The listing builds one solid part. Answer for the finished solid, in the listing's coordinates (mm). A direction names the side the tool comes from. Coordinates: 2 decimals unless noted, no trailing zeros. Loops run counter-clockwise (first coordinate to the right, second up) from the corner with the lowest first, then second, coordinate; pieces in that order, holes last. Notation, with made-up numbers: M 20.25,-18 L 68.25,-18 A19 cw 68.25,-5 Z; hole C 16,-36.75 d10. An arc over 180 degrees is marked long. Answer in a Markdown table with one row per item. Add a question column.
from build123d import *

# Parameters (mm, degrees)
F1_DEPTH = 83.312


with BuildPart() as f1:
    # F0 (on Top) → F1 (new body)
    with BuildSketch(Plane.XY):
        Polygon((3.386476, -29.289481), (23.10539, -18.316191), (29.289481, 3.386476), (18.316191, 23.10539), (-3.386476, 29.289481), (-23.10539, 18.316191), (-29.289481, -3.386476), (-18.316191, -23.10539), align=None)
        Polygon((-15.622193, 7.089933), (-9.309118, 14.410427), (-0.040463, 17.155711), (9.241038, 14.454179), (15.588575, 7.163547), (16.98685, -2.401461), (12.991919, -11.204022), (4.872147, -16.449385), (-4.794498, -16.472184), (-12.938924, -11.265182), (-16.975333, -2.481564), align=None, mode=Mode.SUBTRACT)
    extrude(amount=-F1_DEPTH)


solid = f1.part
(1) A cutting plane is placed at A-A (y = -5.5). Give the vertices of the cut face in (x, z).
(2) A cutting plane is placed at D-D (y = 26). Give the vertices of the cut face in (x, z), plus the area to 3 significant figures.
(3) Each of these flat-tipped pins is pushed along its axis until it touches: pin 1 (2 mm diameter, centred on x = 10.5, z = -11.5, fed in from -Y); pin 2 (10 mm diameter, centred on x = -12.5, z = -29, fed in from +Y); pin 3 (2 mm diameter, centred on y = 15.5, z = -39.5, fed in from -X). Where does it stop, or does it pass through?
(4) The mould has two halves that part along Y. Classify faces 3 (the face through (4.535, 15.824, -41.073)), 4 (the face through (-7.617, -26.154, -41.073)), 5 (the face through (13, -13, 0)): released by +Y, released by -Y, zero draft, split by the parting line, or undercut.
(5) A cutting plane is placed at C-C (x = -1.5). Give the vertices of the cut face in (y, z), plus the area to 3 significant figures.
(6) For faces 1 (the face through (-8.81, -13.905, -41.073)), 2 (the face through (-13.11, 23.88, -41.07)), determine the directions among +Z, -Z, +X, -X, +Y, -Y from which every point of the face is accessible in a straight line to the end or side of a thin tool.
(7) A cutting plane is placed at B-B (z = -38.5). Give the vertices of the cut face in (x, y), plus the area to 3 significant figures.
(8) Straight lines are drawn through the part: line 1 (X direction, y = 3, z = -21.5); line 2 (Y direction, x = -9, z = -47); line 3 (Y direction, x = 0, z = -4.5). For each, find the intervals that lie inside material, in ascending order.
Solved:
| question | item | result |
|---|---|---|
| 1 | outline | M -28.11,-83.31 L -15.59,-83.31 L -15.59,0 L -28.11,0 Z; M 15.58,-83.31 L 26.76,-83.31 L 26.76,0 L 15.58,0 Z |
| 2 | outline | M -9.3,-83.31 L 8.16,-83.31 L 8.16,0 L -9.3,0 Z |
| 2 | area | 1,450 mm² |
| 3 | pin 1 | stops at y = -25.89 |
| 3 | pin 2 | stops at y = 27 |
| 3 | pin 3 | stops at x = -24.19 |
| 4 | face 3 | undercut |
| 4 | face 4 | released by -Y |
| 4 | face 5 | zero draft |
| 5 | outline | M -27.9,-83.31 L -16.46,-83.31 L -16.46,0 L -27.9,0 Z; M 16.72,-83.31 L 28.75,-83.31 L 28.75,0 L 16.72,0 Z |
| 5 | area | 1,950 mm² |
| 6 | face 1 | +Z, -Z |
| 6 | face 2 | +Z, -Z, -X, +Y |
| 7 | outline | M -29.29,-3.39 L -18.32,-23.11 L 3.39,-29.29 L 23.11,-18.32 L 29.29,3.39 L 18.32,23.11 L -3.39,29.29 L -23.11,18.32 Z; hole M -16.98,-2.48 L -12.94,-11.27 L -4.79,-16.47 L 4.87,-16.45 L 12.99,-11.2 L 16.99,-2.4 L 15.59,7.16 L 9.24,14.45 L -0.04,17.16 L -9.31,14.41 L -15.62,7.09 Z |
| 7 | area | 1,580 mm² |
| 8 | line 1 | x = -27.47 to -16.2, 16.2 to 29.18 |
| 8 | line 2 | y = -25.76 to -13.78, 14.5 to 26.17 |
| 8 | line 3 | y = -28.32 to -16.46, 17.14 to 28.32 |
